Part print with two shaded views. Sizes in mm from the minimum x, y, z corner. Round coordinates to 2 decimals unless told otherwise and drop trailing zeros. Write each loop counter-clockwise with the first axis right and the second up, starting at its lowest first coordinate (ties: lowest second). Pieces come first, ordered by that corner, then holes. Notation, with made-up numbers: M 75.5,16.25 L 79.5,16.25 A19 cw 79.5,47.25 Z; hole C 63.5,-26 d6. An arc over 180 degrees is marked long. One line per question, with ' | ' between items. Start each with the question number.
1) Saw through at A-A (y = 35). List the corners of the cut face in (x, z) (1 decimal), plus the area to 3 significant figures.
2) Saw through at B-B (x = 14). List the corners of the cut face in (y, z) (1 decimal), plus the area to 3 significant figures.
3) Saw through at C-C (x = 20.5). List the corners of the cut face in (y, z) (1 decimal).
4) Saw through at D-D (z = 8.75). List the corners of the cut face in (x, y) (1 decimal), plus the area to 3 significant figures.
5) Wall check: probe 1 along Y at (x, z) = (24, 7) (1 decimal); probe 2 along Y at (x, z) = (35.5, 9.5) (1 decimal). Give the ranges that are in metal, low to high. Write a range as [from, to].
6) Mould opens along X. For the marked faces 1, 2 and 3 say: pulls with the +X half, pulls with the -X half, needs draft (parallel to the pull), parting line crosses it, or undercut.
7) Drop flat-ended pins along their axis: pin 1 Ø6 at (x, z) = (38, 10) entering from +Y; pin 2 Ø4 at (x, z) = (25, 10) entering from +Y (1 decimal); pin 3 Ø3 at (x, z) = (7.5, 10) entering from -Y; pin 4 Ø3 at (x, y) = (7.59, 13.83) entering from -Z. Give the stop position or say it passes through.
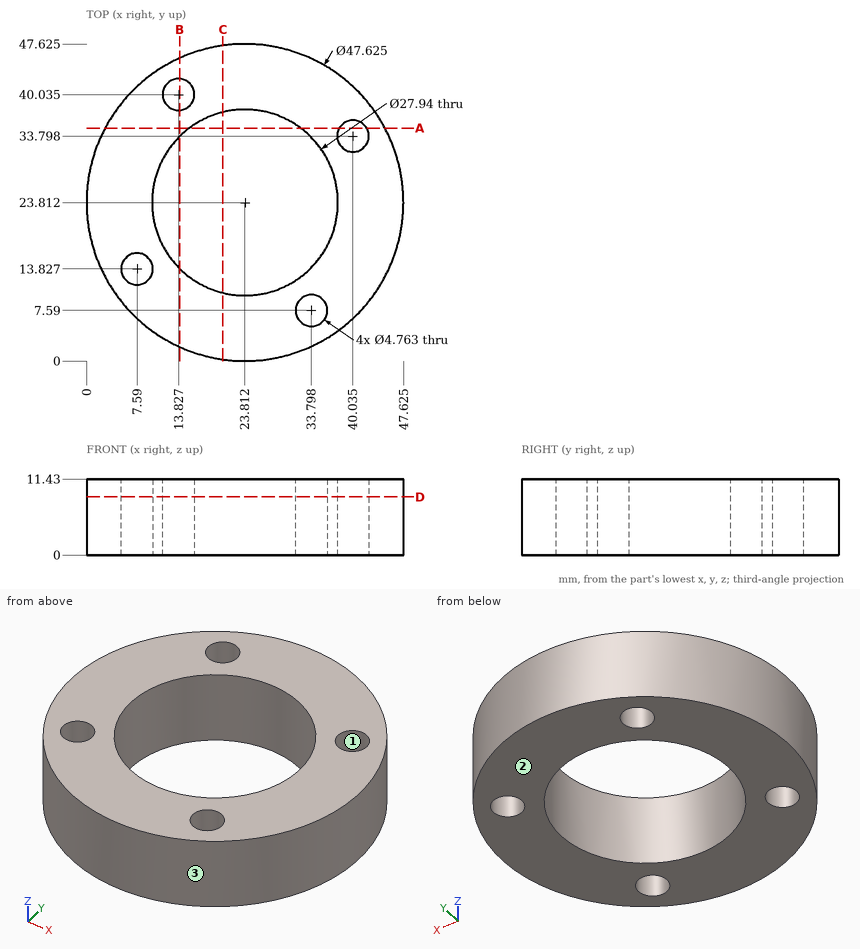
Answer key:
1) outline: M 2.8,0 L 15.4,0 L 15.4,11.4 L 2.8,11.4 Z; M 32.2,0 L 38,0 L 38,11.4 L 32.2,11.4 Z; M 42.1,0 L 44.8,0 L 44.8,11.4 L 42.1,11.4 Z | area: 242 mm2
2) outline: M 2.1,0 L 13.9,0 L 13.9,11.4 L 2.1,11.4 Z; M 33.8,0 L 37.7,0 L 37.7,11.4 L 33.8,11.4 Z; M 42.4,0 L 45.5,0 L 45.5,11.4 L 42.4,11.4 Z | area: 214 mm2
3) outline: M 0.2,0 L 10.2,0 L 10.2,11.4 L 0.2,11.4 Z; M 37.4,0 L 47.4,0 L 47.4,11.4 L 37.4,11.4 Z
4) outline: C 23.8,23.8 d47.6; hole C 7.6,13.8 d4.8; hole C 23.8,23.8 d27.9; hole C 13.8,40 d4.8; hole C 33.8,7.6 d4.8; hole C 40,33.8 d4.8 | area: 1,100 mm2
5) probe 1: y = [0, 9.8], [37.8, 47.6] | probe 2: y = [3.1, 5.9], [9.3, 16.2], [31.5, 44.6]
6) face 1: undercut | face 2: needs draft | face 3: parting line crosses it
7) pin 1: stops at y = 44.83 | pin 2: stops at y = 47.6 | pin 3: stops at y = 5.17 | pin 4: passes through
